Design review of the part built by this model. Coordinates are the model's own, in mm. Face numbers are marked on the shaded views. A direction names the side the tool comes from. Coordinates: 2 decimals unless noted, no trailing zeros. Loops run counter-clockwise (first coordinate to the right, second up) from the corner with the lowest first, then second, coordinate; pieces in that order, holes last. Notation, with made-up numbers: (47.5, -19.5) - (88.5, -19.5) arc R15 ccw to (88.5, 1.5) - close; hole circle Ø5 at (79, -21). An arc over 180 degrees is marked (long way). One line per question, with ' | ' between items.
from build123d import *

# Parameters (mm, degrees)
F0_W     = 151.9381850958
F0_H     = 111.7599979043
F0_R     = 13.8333647365
F0_R_2   = 14.3205526474
F1_DEPTH = 50.8
F3_DEPTH = 25.4
F4_DEPTH = 127
F6_DEPTH = 25.4


with BuildPart() as f1:
    # F0 (on Top) → F1 (new body)
    with BuildSketch(Plane.XY):
        with Locations((-0.2309083939, 0.1154541969)):
            Rectangle(F0_W, F0_H)
        with Locations((-54.7254569829, 0.1154541969)):
            Circle(F0_R, mode=Mode.SUBTRACT)
        with Locations((50.1072742045, 0)):
            Circle(F0_R_2, mode=Mode.SUBTRACT)
    extrude(amount=F1_DEPTH)

    # F2 (on face) → F3 (join)
    with BuildSketch(Plane.XZ.offset(55.7645447552)):
        with BuildLine():
            ThreePointArc((-27.3391341012, 50.8), (-0.2309083939, 23.6917742927), (26.8773173135, 50.8))
            Line((26.8773173135, 50.8), (19.9617576881, 50.8))
            ThreePointArc((19.9617576881, 50.8), (-0.2309083939, 30.6073339181), (-20.4235744758, 50.8))
            Line((-20.4235744758, 50.8), (-27.3391341012, 50.8))
        make_face()
    extrude(amount=F3_DEPTH)

    # F4 (cut): a face of the model
    f4_faces = [f1.faces().sort_by_distance(p)[0] for p in [
        (-0.2309083939, -55.7645447552, 42.2299663436),
    ]]
    extrude(f4_faces, amount=-F4_DEPTH, mode=Mode.SUBTRACT)

    # F5 (on face) → F6 (join)
    with BuildSketch(Plane(origin=(0, 55.9954531491, 0), x_dir=(-1, 0, 0), z_dir=(0, 1, 0))):
        with BuildLine():
            ThreePointArc((-27.1668712907, 50.8), (0.2309083939, 23.4022203155), (27.6286880784, 50.8))
            Line((27.6286880784, 50.8), (20.4235744758, 50.8))
            ThreePointArc((20.4235744758, 50.8), (0.2309083939, 30.6073339181), (-19.9617576881, 50.8))
            Line((-19.9617576881, 50.8), (-27.1668712907, 50.8))
        make_face()
    extrude(amount=F6_DEPTH)


solid = f1.part
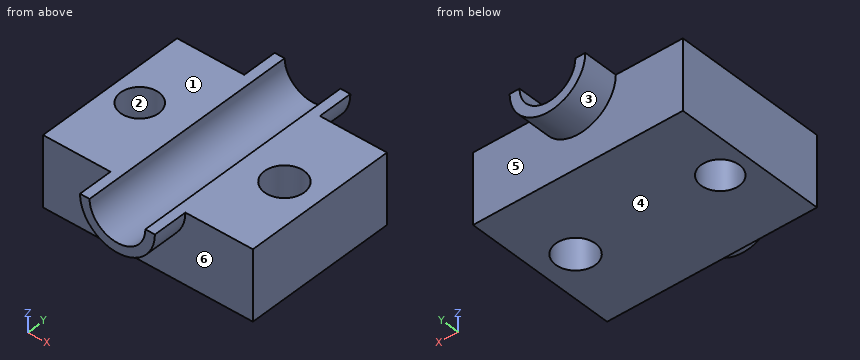
Q1. Tool access review of the marked faces 4, 5 and 6: name each direction out of +Z, -Z, +X, -X, +Y, -Y from which nothing blocks a thin tool from reaching the whole face with its end or side.
Returned:
face 4: -Z, +X, -X, +Y, -Y | face 5: -Z, +Y | face 6: -Z, -Y
Q2. Take a section at B-B (x = -65). Give the boundary of the cut face in (y, z), plus the area to 3 significant figures.
Returned:
outline: (-55.76, 0) - (-9.15, 0) - (-9.15, 50.8) - (-55.76, 50.8) - close; (9.38, 0) - (56, 0) - (56, 50.8) - (9.38, 50.8) - close | area: 4,740 mm²
Q3. Take a section at C-C (y = 12). Give the boundary of the cut face in (x, z).
Returned:
outline: (-76.2, 0) - (-61.8, 0) - (-61.8, 50.8) - (-76.2, 50.8) - close; (-47.65, 0) - (42.29, 0) - (42.29, 50.8) - (19.96, 50.8) arc R20.19 cw to (-20.42, 50.8) - (-47.65, 50.8) - close; (57.92, 0) - (75.74, 0) - (75.74, 50.8) - (57.92, 50.8) - close
Q4. Take a section at D-D (z = 35). Give the boundary of the cut face in (x, y).
Returned:
outline: (-76.2, -55.76) - (-22.26, -55.76) - (-22.26, -81.16) - (-12.8, -81.16) - (-12.8, 81.4) - (-22.61, 81.4) - (-22.61, 56) - (-76.2, 56) - close; (12.34, -81.16) - (21.8, -81.16) - (21.8, -55.76) - (75.74, -55.76) - (75.74, 56) - (22.15, 56) - (22.15, 81.4) - (12.34, 81.4) - close; hole circle Ø27.67 at (-54.73, 0.12); hole circle Ø28.64 at (50.11, 0)
Q5. To check wall thickness, follow line 1 along X through (y, z) = (-9.5, 23.5); line 2 along X through (y, z) = (-6, 30.5); line 3 along X through (y, z) = (43, 36). State the ranges of each line that lie inside material, in increasing order.
Returned:
line 1: x = -76.2 to -64.67, -44.78 to 39.39, 60.82 to 75.74 | line 2: x = -76.2 to -67.13, -42.32 to 37.1, 63.11 to 75.74 | line 3: x = -76.2 to -13.97, 13.51 to 75.74
Q6. Draft analysis for pull direction X (two halves, no side actions). For the marked faces 1, 2 and 3, state which applies: +X half, -X half, draft (parallel to the pull), parting line (faces both ways), or undercut.
Returned:
face 1: draft | face 2: undercut | face 3: parting line
Q7. Take a section at A-A (z = 43.5). Give the boundary of the cut face in (x, y).
Returned:
outline: (-76.2, -55.76) - (-26.34, -55.76) - (-26.34, -81.16) - (-19.06, -81.16) - (-19.06, 81.4) - (-26.64, 81.4) - (-26.64, 56) - (-76.2, 56) - close; (18.6, -81.16) - (25.88, -81.16) - (25.88, -55.76) - (75.74, -55.76) - (75.74, 56) - (26.18, 56) - (26.18, 81.4) - (18.6, 81.4) - close; hole circle Ø27.67 at (-54.73, 0.12); hole circle Ø28.64 at (50.11, 0)
Q8. For pin 1 (10 mm diameter, centred on x = -51.5, z = 30, fed in from -Y); pin 2 (10 mm diameter, centred on x = 8.5, y = -11, fed in from -Z); pin 3 (4 mm diameter, centred on x = -40, z = 35, fed in from +Y), all flat-tipped, find the tip position at first contact; note any pin that passes through.
Returned:
pin 1: stops at y = -55.76 | pin 2: stops at z = 0 | pin 3: stops at y = 56
